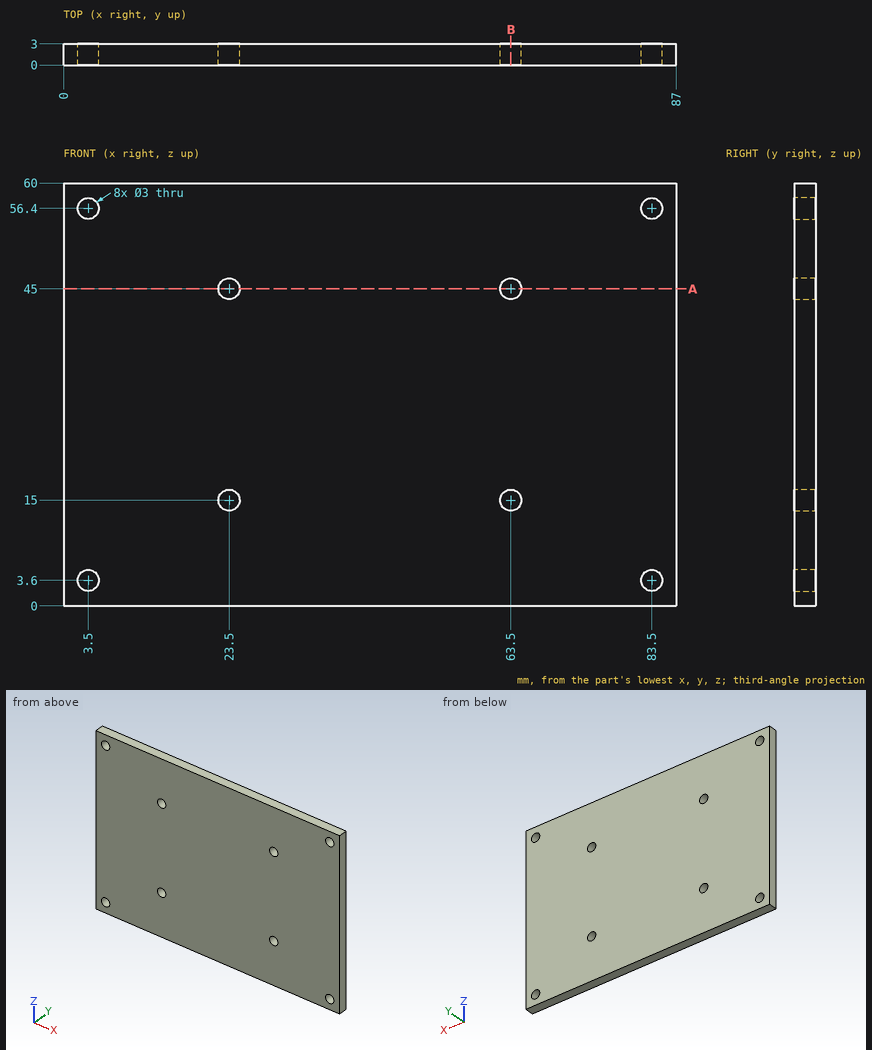
Geometry check sheet. Reference: drawing and pictorial views, mm from the part's lowest x, y, z. Round coordinates to 2 decimals unless told otherwise and drop trailing zeros. Loops run counter-clockwise (first coordinate to the right, second up) from the corner with the lowest first, then second, coordinate; pieces in that order, holes last.
1. Sectioned sample at A-A on z = 45. Record the boundary of the cut face in (x, y), and give its area (3 significant figures).
2. Scan lines: probe 1 along X at (y, z) = (1.1, 45); probe 2 along X at (y, z) = (1.6, 56.4); probe 3 along Z at (x, y) = (64.5, 0.4). Record each from-to range of solid material in increasing order.
3. Sectioned sample at B-B on x = 63.5. Record the boundary of the cut face in (y, z).
4. Gauge pin test, flat end, axial feed: pin 1 Ø2.5 at (x, z) = (63.5, 15) entering from +Y. Record the tip position at first contact, or that the pin passes through.
Recorded:
1. outline: (0, 0) - (22, 0) - (22, 3) - (0, 3) - close; (25, 0) - (62, 0) - (62, 3) - (25, 3) - close; (65, 0) - (87, 0) - (87, 3) - (65, 3) - close
1. area: 243 mm2
2. probe 1: x = 0 to 22, 25 to 62, 65 to 87
2. probe 2: x = 0 to 2, 5 to 82, 85 to 87
2. probe 3: z = 0 to 13.88, 16.12 to 43.88, 46.12 to 60
3. outline: (0, 0) - (3, 0) - (3, 13.5) - (0, 13.5) - close; (0, 16.5) - (3, 16.5) - (3, 43.5) - (0, 43.5) - close; (0, 46.5) - (3, 46.5) - (3, 60) - (0, 60) - close
4. pin 1: passes through
